```python
from build123d import *

# Parameters (mm, degrees)
SKETCH1_W           = 170
SKETCH1_H           = 240
BOSS_EXTRUDE1_DEPTH = 5
SKETCH2_R           = 16.5
CUT_EXTRUDE1_DEPTH  = 148.139389696
SKETCH3_R           = 2
CUT_EXTRUDE2_DEPTH  = 148.139389696
SKETCH4_R           = 1.7
CUT_EXTRUDE3_DEPTH  = 148.139389696
SKETCH5_W           = 75
SKETCH5_H           = 35
CUT_EXTRUDE4_DEPTH  = 148.139389696
FILLET1_R           = 4
SKETCH6_R           = 2.000000001
CUT_EXTRUDE5_DEPTH  = 148.139389696
FILLET2_R           = 4
SKETCH7_R           = 2.5
CUT_EXTRUDE6_DEPTH  = 148.139389696
SKETCH8_R           = 2.5
CUT_EXTRUDE7_DEPTH  = 148.139389696


with BuildPart() as part:
    # Sketch1 → Boss-Extrude1 (new body)
    with BuildSketch(Plane.XY):
        Rectangle(SKETCH1_W, SKETCH1_H)
    extrude(amount=BOSS_EXTRUDE1_DEPTH)

    # Sketch2 → Cut-Extrude1 (cut, through all)
    with BuildSketch(Plane.XY.offset(5)):
        with Locations((62.5, 0)):
            Circle(SKETCH2_R)
    extrude(amount=-CUT_EXTRUDE1_DEPTH, mode=Mode.SUBTRACT)

    # Sketch3 → Cut-Extrude2 (cut, through all)
    with BuildSketch(Plane.XY.offset(5)):
        with Locations((72.5, -17.320508076)):
            Circle(SKETCH3_R)
        with Locations((72.5, 17.320508076)):
            Circle(SKETCH3_R)
        with Locations((42.5, 0)):
            Circle(SKETCH3_R)
    extrude(amount=-CUT_EXTRUDE2_DEPTH, mode=Mode.SUBTRACT)

    # Sketch4 → Cut-Extrude3 (cut, through all)
    with BuildSketch(Plane.XY.offset(5)):
        with Locations((-25, 47)):
            Circle(SKETCH4_R)
        with Locations((-25, 71)):
            Circle(SKETCH4_R)
        with Locations((-55, 47)):
            Circle(SKETCH4_R)
        with Locations((-55, 71)):
            Circle(SKETCH4_R)
        with Locations(Location((-55, -71, 0), (0, 0, 180))):
            Circle(SKETCH4_R)
        with Locations(Location((-25, -71, 0), (0, 0, 180))):
            Circle(SKETCH4_R)
        with Locations(Location((-55, -47, 0), (0, 0, 180))):
            Circle(SKETCH4_R)
        with Locations(Location((-25, -47, 0), (0, 0, 180))):
            Circle(SKETCH4_R)
    extrude(amount=-CUT_EXTRUDE3_DEPTH, mode=Mode.SUBTRACT)

    # Sketch5 → Cut-Extrude4 (cut, through all)
    with BuildSketch(Plane.XY.offset(5)):
        with Locations((-47.5, 102.5)):
            Rectangle(SKETCH5_W, SKETCH5_H)
        with Locations((-47.5, -102.5)):
            Rectangle(SKETCH5_W, SKETCH5_H)
    extrude(amount=-CUT_EXTRUDE4_DEPTH, mode=Mode.SUBTRACT)

    # Fillet1
    fillet1_edges = [part.edges().sort_by_distance(p)[0] for p in [
        (85, -120, 2.5),
    ]]
    fillet(fillet1_edges, radius=FILLET1_R)

    # Sketch6 → Cut-Extrude5 (cut, through all)
    with BuildSketch(Plane.XY.offset(5)):
        with Locations((81.999999999, -117)):
            Circle(SKETCH6_R)
    cut_extrude5 = extrude(amount=-CUT_EXTRUDE5_DEPTH, mode=Mode.SUBTRACT)

    # Mirror5: Cut-Extrude5 across plane
    add(cut_extrude5.mirror(Plane.ZX), mode=Mode.SUBTRACT)

    # Fillet2
    fillet2_edges = [part.edges().sort_by_distance(p)[0] for p in [
        (85, 120, 2.5),
    ]]
    fillet(fillet2_edges, radius=FILLET2_R)

    # Sketch7 → Cut-Extrude6 (cut, through all)
    with BuildSketch(Plane.XY.offset(5)):
        with Locations((41.7, 107.25)):
            Circle(SKETCH7_R)
        with Locations((41.7, 67.25)):
            Circle(SKETCH7_R)
        with Locations((1.7, 67.25)):
            Circle(SKETCH7_R)
        with Locations((1.7, 107.25)):
            Circle(SKETCH7_R)
        with Locations((41.7, -107.25)):
            Circle(SKETCH7_R)
        with Locations((1.7, -107.25)):
            Circle(SKETCH7_R)
        with Locations((1.7, -67.25)):
            Circle(SKETCH7_R)
        with Locations((41.7, -67.25)):
            Circle(SKETCH7_R)
    extrude(amount=-CUT_EXTRUDE6_DEPTH, mode=Mode.SUBTRACT)

    # Sketch8 → Cut-Extrude7 (cut, through all)
    with BuildSketch(Plane(origin=(0, 0, 0), x_dir=(-1, 0, 0), z_dir=(0, 0, -1))):
        with Locations((-63, 106)):
            Circle(SKETCH8_R)
        with Locations((-63, -106)):
            Circle(SKETCH8_R)
        with Locations((70, 0)):
            Circle(SKETCH8_R)
    extrude(amount=-CUT_EXTRUDE7_DEPTH, mode=Mode.SUBTRACT)


solid = part.part
```
Can you work these out from the model? Positions are in its coordinate system, mm. A direction names the side the tool comes from. Coordinates: 2 decimals unless noted, no trailing zeros. Order: outer loops, then holes, each group sorted by start corner. A loop starts at its lowest first (then second) coordinate and runs counter-clockwise, first axis right, second up. Notation, with made-up numbers: (35, 50.5) - (66, 50.5) arc R26 cw to (66, 88.5) - close; hole circle Ø5 at (71.25, 3). An arc over 180 degrees is marked (long way). Answer in a Markdown table with one row per item.
1. Suppose I cut it at D-D (z = 4.05). Give the number of separate pieces and of enclosed holes in the cut face, and give its area (3 significant figures).
Reply:
| item | result |
|---|---|
| separate pieces | 1 |
| enclosed holes | 25 |
| area | 34,300 mm^2 |
2. If I drill on line 1 along X through (y, z) = (71, 1.9); line 2 along Y through (x, z) = (-25, 2.75); line 3 along Y through (x, z) = (1.7, 3), over which ranges is the centre line in solid material (lowest first)?
Reply:
| item | result |
|---|---|
| line 1 | x = -85 to -56.7, -53.3 to -26.7, -23.3 to 85 |
| line 2 | y = -85 to -72.7, -69.3 to -48.7, -45.3 to 45.3, 48.7 to 69.3, 72.7 to 85 |
| line 3 | y = -120 to -109.75, -104.75 to -69.75, -64.75 to 64.75, 69.75 to 104.75, 109.75 to 120 |
3. If we mould it in two halves opening along Y, with no side actions, what happens to faces 4 (the cylindrical face through (39.202, 67.36, 2.535)), 5 (the flat face through (35, -120, 2)), 6 (the flat face through (-10, 102, 3))? For each: pulls with the +Y half, pulls with the -Y half, needs draft (parallel to the pull), parting line crosses it, or undercut.
Reply:
| item | result |
|---|---|
| face 4 | undercut |
| face 5 | pulls with the -Y half |
| face 6 | needs draft |
4. Suppose I cut it at B-B (x = 63). Please give me the cut outline in (y, z), and give its area (3 significant figures).
Reply:
| item | result |
|---|---|
| outline | (-120, 0) - (-108.5, 0) - (-108.5, 5) - (-120, 5) - close; (-103.5, 0) - (-16.49, 0) - (-16.49, 5) - (-103.5, 5) - close; (16.49, 0) - (103.5, 0) - (103.5, 5) - (16.49, 5) - close; (108.5, 0) - (120, 0) - (120, 5) - (108.5, 5) - close |
| area | 985 mm^2 |
5. Suppose I cut it at C-C (y = -89.5). Please give me the cut outline in (x, z), and give its area (3 significant figures).
Reply:
| item | result |
|---|---|
| outline | (-10, 0) - (85, 0) - (85, 5) - (-10, 5) - close |
| area | 475 mm^2 |
6. Suppose I cut it at A-A (x = -70). Please give me the cut outline in (y, z).
Reply:
| item | result |
|---|---|
| outline | (-85, 0) - (-2.5, 0) - (-2.5, 5) - (-85, 5) - close; (2.5, 0) - (85, 0) - (85, 5) - (2.5, 5) - close |
7. For faces 1 (the flat face through (-48, 85, 3)), 2 (the cylindrical face through (39.202, 107.36, 2.535)), 3 (the flat face through (-48, -85, 3)), which set-ups out of +Z, -Z, +X, -X, +Y, -Y let a thin tool reach every point of the face, with its end or its side?
Reply:
| item | result |
|---|---|
| face 1 | +Z, -Z, -X, +Y |
| face 2 | +Z, -Z |
| face 3 | +Z, -Z, -X, -Y |
8. For pin 1 (2 mm diameter, centred on x = -36.5, z = 4.5, fed in from -Y); pin 2 (2.5 mm diameter, centred on x = 72.5, y = 17.32, fed in from +Z); pin 3 (2.5 mm diameter, centred on y = 96, z = 1.5, fed in from -X), each with a flat end and sliding along its axis, tell me the tip position at first contact or that it passes through.
Reply:
| item | result |
|---|---|
| pin 1 | stops at y = -85 |
| pin 2 | passes through |
| pin 3 | stops at x = -10 |
